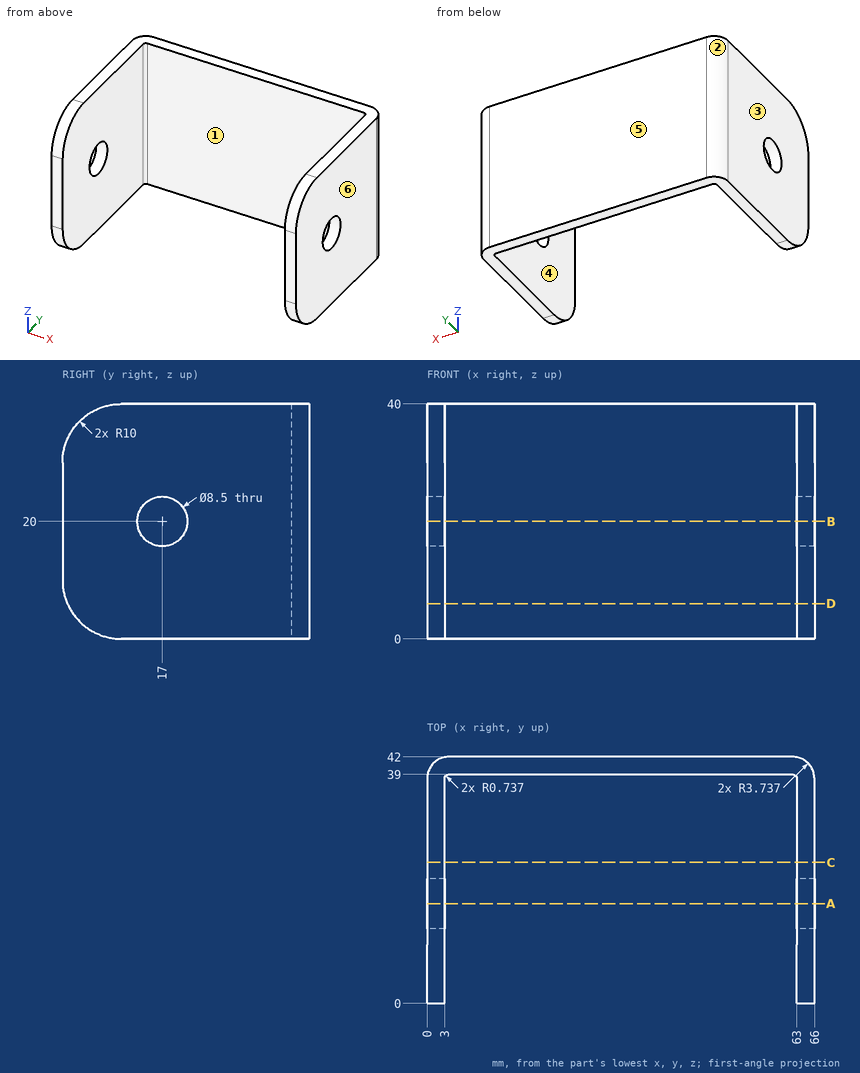
Design review of the part shown in the three views and the two pictorial views. Dimensions are in mm from the part's minimum x, y and z. A direction names the side the tool comes from. Give positions to 0.01 mm unless a question says otherwise; leave off trailing zeros. Loops run counter-clockwise (first coordinate to the right, second up) from the corner with the lowest first, then second, coordinate; pieces in that order, holes last. Notation, with made-up numbers: (82.5, 19.5) -> (93.5, 19.5) arc R7 ccw to (93.5, 30.5) -> close; hole circle Ø8 at (36, -3). An arc over 180 degrees is marked (long way). Put each result on its own line as item: value. Start each with the question number.
1. We need section D-D on z = 6. State the section outline as (x, y) points (1 decimal).
2. We need section A-A on y = 17. State the section outline as (x, z) points, then the cut area to 3 significant figures.
3. Clearance check with a flat-ended pin moving along its axis: P1, Ø1, axis at x = 47, z = 20, coming from the -Y side. State where the tip first meets the part, or that it passes through.
4. We need section B-B on z = 20. State the section outline as (x, y) points, then the cut area to 3 significant figures.
5. Mouldability with a two-part tool opening along X and no side actions: class the marked faces 3, 4, 5 and 6 as released by +X, released by -X, zero draft, split by the parting line, or undercut.
6. Wall thickness on probe 1 along X at (y, z) = (29, 16.5); probe 2 along Y at (x, z) = (62, 35); probe 3 along Y at (x, z) = (0.75, 20): over which ranges is each line inside the solid? List them lowest first.
7. For the marked faces 1 and 2, list the 3-axis set-ups (+Z, -Z, +X, -X, +Y, -Y) from which the entire face can be reached by the end or side of a thin tool; tool diameter is ignored.
8. We need section C-C on y = 24. State the section outline as (x, z) points.
Determined:
1. outline: (0, 0.8) -> (3, 0.8) -> (3, 38.3) arc R0.7 cw to (3.7, 39) -> (62.3, 39) arc R0.7 cw to (63, 38.3) -> (63, 0.8) -> (66, 0.8) -> (66, 38.3) arc R3.7 ccw to (62.3, 42) -> (3.7, 42) arc R3.7 ccw to (0, 38.3) -> close
2. outline: (0, 0) -> (3, 0) -> (3, 15.75) -> (0, 15.75) -> close; (0, 24.25) -> (3, 24.25) -> (3, 40) -> (0, 40) -> close; (63, 0) -> (66, 0) -> (66, 15.75) -> (63, 15.75) -> close; (63, 24.25) -> (66, 24.25) -> (66, 40) -> (63, 40) -> close
2. area: 189 mm^2
3. P1: y = 39
4. outline: (0, 0) -> (3, 0) -> (3, 12.75) -> (0, 12.75) -> close; (0, 21.25) -> (3, 21.25) -> (3, 38.26) arc R0.74 cw to (3.74, 39) -> (62.26, 39) arc R0.74 cw to (63, 38.26) -> (63, 21.25) -> (66, 21.25) -> (66, 38.26) arc R3.74 ccw to (62.26, 42) -> (3.74, 42) arc R3.74 ccw to (0, 38.26) -> close; (63, 0) -> (66, 0) -> (66, 12.75) -> (63, 12.75) -> close
4. area: 375 mm^2
5. face 3: released by -X
5. face 4: undercut
5. face 5: zero draft
5. face 6: released by +X
6. probe 1: 0 to 3, 63 to 66
6. probe 2: 39 to 42
6. probe 3: 0 to 12.75, 21.25 to 40.51
7. face 1: +Z, -Z, -Y
7. face 2: +Z, -Z, -X, +Y
8. outline: (0, 0) -> (3, 0) -> (3, 40) -> (0, 40) -> close; (63, 0) -> (66, 0) -> (66, 40) -> (63, 40) -> close
